Here's how the part is built. I have some questions about the finished solid (model axes, mm). A direction names the side the tool comes from. Round coordinates to 2 decimals unless told otherwise and drop trailing zeros. Loops run counter-clockwise (first coordinate to the right, second up) from the corner with the lowest first, then second, coordinate; pieces in that order, holes last. Notation, with made-up numbers: M -22,64.5 L -13,64.5 A6 cw -13,70.5 Z; hole C 76,-15 d9. An arc over 180 degrees is marked long. Put each result on its own line as item: value. Start each with the question number.
```python
from build123d import *

# Parameters (mm, degrees)
F1_DEPTH = 6
F2_W     = 10
F2_H     = 6
F3_DEPTH = 25


with BuildPart() as f1:
    # F0 (on Front) → F1 (new body)
    with BuildSketch(Plane.XZ):
        with BuildLine():
            Line((80, 132), (-80, 132))
            Line((-80, 132), (-80, 117))
            Line((-80, 117), (-80, 102))
            Line((-80, 102), (-80, 74.330344))
            ThreePointArc((-80, 74.330344), (-77.527727, 67.747538), (-71.333333, 64.419631))
            ThreePointArc((-71.333333, 64.419631), (-15, 0), (-71.333333, -64.419631))
            ThreePointArc((-71.333333, -64.419631), (-77.527727, -67.747538), (-80, -74.330344))
            Line((-80, -74.330344), (-80, -102))
            Line((-80, -102), (-80, -117))
            Line((-80, -117), (-80, -132))
            Line((-80, -132), (-74.330344, -132))
            ThreePointArc((-74.330344, -132), (-67.747538, -129.527727), (-64.419631, -123.333333))
            ThreePointArc((-64.419631, -123.333333), (0, -67), (64.419631, -123.333333))
            ThreePointArc((64.419631, -123.333333), (67.747538, -129.527727), (74.330344, -132))
            Line((74.330344, -132), (80, -132))
            Line((80, -132), (80, -117))
            Line((80, -117), (80, -102))
            Line((80, -102), (80, -74.330344))
            ThreePointArc((80, -74.330344), (77.527727, -67.747538), (71.333333, -64.419631))
            ThreePointArc((71.333333, -64.419631), (15, 0), (71.333333, 64.419631))
            ThreePointArc((71.333333, 64.419631), (77.527727, 67.747538), (80, 74.330344))
            Line((80, 74.330344), (80, 102))
            Line((80, 102), (80, 117))
            Line((80, 117), (80, 132))
        make_face()
        with BuildLine():
            Line((-80, 102), (-80, 117))
            Line((-80, 117), (-99, 117))
            ThreePointArc((-99, 117), (-100.414214, 116.414214), (-101, 115))
            Line((-101, 115), (-101, 104))
            ThreePointArc((-101, 104), (-100.414214, 102.585786), (-99, 102))
            Line((-99, 102), (-80, 102))
        make_face()
        with BuildLine():
            Line((99, 117), (80, 117))
            Line((80, 117), (80, 102))
            Line((80, 102), (99, 102))
            ThreePointArc((99, 102), (100.414214, 102.585786), (101, 104))
            Line((101, 104), (101, 115))
            ThreePointArc((101, 115), (100.414214, 116.414214), (99, 117))
        make_face()
        with BuildLine():
            Line((-80, -117), (-80, -102))
            Line((-80, -102), (-99, -102))
            ThreePointArc((-99, -102), (-100.414214, -102.585786), (-101, -104))
            Line((-101, -104), (-101, -115))
            ThreePointArc((-101, -115), (-100.414214, -116.414214), (-99, -117))
            Line((-99, -117), (-80, -117))
        make_face()
        with BuildLine():
            Line((99, -102), (80, -102))
            Line((80, -102), (80, -117))
            Line((80, -117), (99, -117))
            ThreePointArc((99, -117), (100.414214, -116.414214), (101, -115))
            Line((101, -115), (101, -104))
            ThreePointArc((101, -104), (100.414214, -102.585786), (99, -102))
        make_face()
    extrude(amount=F1_DEPTH)

    # F2 (on face) → F3 (cut)
    with BuildSketch(Plane.XZ.offset(6)):
        with Locations((-90, 109.5)):
            Rectangle(F2_W, F2_H)
        with Locations((90, 109.5)):
            Rectangle(F2_W, F2_H)
        with Locations((-90, -109.5)):
            Rectangle(F2_W, F2_H)
        with Locations((90, -109.5)):
            Rectangle(F2_W, F2_H)
    extrude(amount=-F3_DEPTH, mode=Mode.SUBTRACT)


solid = f1.part
```
1) If we mould it in two halves opening along Z, with no side actions, what happens to faces 4 (the face through (77, -3, -132)), 5 (the face through (90, -3, 117)), 6 (the face through (89, -3, 102))? For each: pulls with the +Z half, pulls with the -Z half, needs draft (parallel to the pull), parting line crosses it, or undercut.
2) On a 3-axis mill with a long thin cutter (end or side, diameter ignored), from which of +Z, -Z, +X, -X, +Y, -Y can I reach the whole of each face in a straight line? I mean faces 1 (the face through (-77.46, -2.96, -67.67)), 2 (the face through (-89, -3, 117)), 3 (the face through (89, -3, -117)). Say none if no direction works.
3) Suppose I cut it at C-C (z = -85). Write out the boundary of the cut face in (x, y), plus the area to 3 significant figures.
4) If I drill on probe 1 along Z at (x, y) = (91, -3.95); probe 2 along X at (y, z) = (-2.2, -111.5); probe 3 along X at (y, z) = (-1.35, 75), over which ranges is the centre line in solid material (lowest first)? Write a range as from..to.
5) I'm going to push flat-ended pins straight in: P1, Ø1.5, axis at y = -2, z = 100, coming from the -X side; P2, Ø1.5, axis at x = 18, z = 7, coming from the -Y side; P3, Ø1.8, axis at y = -2.5, z = -91.5, coming from the +X side; P4, Ø3, axis at x = 90, y = -2.5, coming from the +Z side. Where does each tip first touch, or does it pass through?
6) Suppose I cut it at B-B (x = 21.5). Write out the boundary of the cut face in (y, z), plus the area to 3 significant figures.
7) Suppose I cut it at A-A (x = -88.5). Write out the boundary of the cut face in (y, z).
8) Suppose I cut it at D-D (z = 80). Write out the boundary of the cut face in (x, y), plus the area to 3 significant figures.
Results are:
1. face 4: pulls with the -Z half
1. face 5: pulls with the +Z half
1. face 6: undercut
2. face 1: -X, +Y, -Y
2. face 2: +Z, -X, +Y, -Y
2. face 3: -Z, +X, +Y, -Y
3. outline: M -80,-6 L -44.9,-6 L -44.9,0 L -80,0 Z; M 44.9,-6 L 80,-6 L 80,0 L 44.9,0 Z
3. area: 421 mm²
4. probe 1: -117..-112.5, -106.5..-102, 102..106.5, 112.5..117
4. probe 2: -101..-95, -85..-61.68, 61.68..85, 95..101
4. probe 3: -80..80
5. P1: x = -80
5. P2: through
5. P3: x = 80
5. P4: z = 117
6. outline: M -6,-70.66 L 0,-70.66 L 0,-28.33 L -6,-28.33 Z; M -6,28.33 L 0,28.33 L 0,132 L -6,132 Z
6. area: 876 mm²
7. outline: M -6,-117 L 0,-117 L 0,-112.5 L -6,-112.5 Z; M -6,-106.5 L 0,-106.5 L 0,-102 L -6,-102 Z; M -6,102 L 0,102 L 0,106.5 L -6,106.5 Z; M -6,112.5 L 0,112.5 L 0,117 L -6,117 Z
8. outline: M -80,-6 L 80,-6 L 80,0 L -80,0 Z
8. area: 960 mm²
